Read the model definition and answer for the solid it produces. Units are mm, in the model's axes. Face numbers are marked on the shaded views. A direction names the side the tool comes from. Coordinates: 2 decimals unless noted, no trailing zeros. Write each loop counter-clockwise with the first axis right and the second up, starting at its lowest first coordinate (ties: lowest second). Pieces come first, ordered by that corner, then holes. Notation, with made-up numbers: (47.25, -23.75) -> (67.25, -23.75) arc R19 cw to (67.25, 0.25) -> close; hole circle Ø8 at (0.5, 56). An arc over 180 degrees is marked (long way). Answer as a JSON object with one key per item and string values. Group by question number.
(1) Find section D-D (y = -24). Give the vertices of the cut face in (x, z).
(2) For a pull along Y with two mould halves and no side action, classify the marked faces 1, 2 and 3 as +Y half, -Y half, draft (parallel to the pull), parting line (faces both ways), or undercut.
(3) Flat-ended cylindrical pins translate along their axes: P1, Ø10, axis at y = 10, z = 11, coming from the +X side; P2, Ø3, axis at x = 34, y = 0, coming from the +Z side; P3, Ø6, axis at y = -68.5, z = 5.5, coming from the +X side; P4, Ø1.5, axis at y = -61.5, z = 13, coming from the +X side. Find the tip coordinate at first contact, or state that the pin passes through.
(4) Find section A-A (z = -9). Give the vertices of the cut face in (x, y).
(5) Find section B-B (y = -65.5). Give the vertices of the cut face in (x, z), then the cut area to 3 significant figures.
(6) Straight lines are drawn through the part: L1, parallel to Y at x = 14.5, z = -5; L2, parallel to Y at x = -17, z = 12.5; L3, parallel to Y at x = -17, z = 8.25. For each, find the intervals that lie inside material, in ascending order.
(7) Which of the six approach directions +Z, -Z, +X, -X, +Y, -Y give full straight-line access (tool end or side, diameter ignored) to the marked faces 4, 5, 6, 7 and 8?
(8) Find section C-C (z = 2). Give the vertices of the cut face in (x, y), then the cut area to 3 significant figures.
from build123d import *

# Parameters (mm, degrees)
SKETCH1_R               = 37.5
SKETCH1_R_2             = 29.5
BOSS_EXTRUDE1_DEPTH     = 15
SKETCH2_R               = 32.5
SKETCH2_R_2             = 27.5
CUT_EXTRUDE1_DEPTH      = 7
SKETCH9_R               = 1
CUT_EXTRUDE5_DEPTH      = 15
SKETCH10_R              = 37.5
CUT_EXTRUDE6_DEPTH      = 4
SKETCH7_W               = 45
SKETCH7_H               = 10
BOSS_EXTRUDE3_DEPTH     = 12.5
SKETCH12_R              = 1.5
CUT_EXTRUDE8_DEPTH      = 15
CUT_EXTRUDE9_DEPTH      = 35
CUT_EXTRUDE9_DEPTH_BACK = 35
SKETCH14_W              = 8
SKETCH14_H              = 44.996878368
CUT_EXTRUDE10_DEPTH     = 5


with BuildPart() as part:
    # Sketch1 → Boss-Extrude1 (new body)
    # profile 1 of 2: a face of its own
    with BuildSketch(Plane.XY):
        Circle(SKETCH1_R)
        Circle(SKETCH1_R_2, mode=Mode.SUBTRACT)
    # profile 2 of 2: a face of its own
    with BuildSketch(Plane.XY):
        with BuildLine():
            Line((-22.5, -82.5), (22.5, -82.5))
            Line((22.5, -82.5), (36.841286084, -6.997831068))
            ThreePointArc((36.841286084, -6.997831068), (0, -37.5), (-36.841286084, -6.997831068))
            Line((-36.841286084, -6.997831068), (-22.5, -82.5))
        make_face()
    extrude(amount=BOSS_EXTRUDE1_DEPTH)

    # Sketch2 → Cut-Extrude1 (cut)
    with BuildSketch(Plane(origin=(0, 0, 0), x_dir=(-1, 0, 0), z_dir=(0, 0, -1))):
        Circle(SKETCH2_R)
        Circle(SKETCH2_R_2, mode=Mode.SUBTRACT)
    extrude(amount=-CUT_EXTRUDE1_DEPTH, mode=Mode.SUBTRACT)

    # Sketch9 → Cut-Extrude5 (cut)
    with BuildSketch(Plane.XY.offset(15)):
        with Locations((17, 29.444863729)):
            Circle(SKETCH9_R)
        with Locations((34, 0)):
            Circle(SKETCH9_R)
        with Locations((17, -29.444863729)):
            Circle(SKETCH9_R)
        with Locations((-17, -29.444863729)):
            Circle(SKETCH9_R)
        with Locations((-34, 0)):
            Circle(SKETCH9_R)
        with Locations((-17, 29.444863729)):
            Circle(SKETCH9_R)
    extrude(amount=-CUT_EXTRUDE5_DEPTH, mode=Mode.SUBTRACT)

    # Sketch10 → Cut-Extrude6 (cut)
    with BuildSketch(Plane(origin=(0, 0, 0), x_dir=(-1, 0, 0), z_dir=(0, 0, -1))):
        Circle(SKETCH10_R)
    extrude(amount=-CUT_EXTRUDE6_DEPTH, mode=Mode.SUBTRACT)

    # Sketch7 → Boss-Extrude3 (add)
    with BuildSketch(Plane(origin=(0, 0, 0), x_dir=(-1, 0, 0), z_dir=(0, 0, -1))):
        with Locations((0, -77.5)):
            Rectangle(SKETCH7_W, SKETCH7_H)
        with Locations((0, -42.5)):
            Rectangle(SKETCH7_W, SKETCH7_H)
    extrude(amount=BOSS_EXTRUDE3_DEPTH)

    # Sketch12 → Cut-Extrude8 (cut)
    with BuildSketch(Plane(origin=(0, 0, 0), x_dir=(-1, 0, 0), z_dir=(0, 0, -1))):
        with Locations((-15, -54.5)):
            Circle(SKETCH12_R)
        with Locations((0, -54.5)):
            Circle(SKETCH12_R)
        with Locations((15, -54.5)):
            Circle(SKETCH12_R)
        with Locations((-15, -65.5)):
            Circle(SKETCH12_R)
        with Locations((0, -65.5)):
            Circle(SKETCH12_R)
        with Locations((15, -65.5)):
            Circle(SKETCH12_R)
    extrude(amount=-CUT_EXTRUDE8_DEPTH, mode=Mode.SUBTRACT)

    # Sketch13 → Cut-Extrude9 (cut, two sides: drawn at the far end of the back side and taken through both)
    with BuildSketch(Plane(origin=(0, 0, 0), x_dir=(0, 0, -1), z_dir=(1, 0, 0)).offset(-CUT_EXTRUDE9_DEPTH_BACK)):
        Polygon((-15, -82.5), (-15, -37.5), (-10, -82.5), align=None)
    extrude(amount=CUT_EXTRUDE9_DEPTH + CUT_EXTRUDE9_DEPTH_BACK, mode=Mode.SUBTRACT)

    # Sketch14 → Cut-Extrude10 (cut)
    with BuildSketch(Plane.XY.offset(15)):
        with Locations((-15, -59.998439184)):
            Rectangle(SKETCH14_W, SKETCH14_H)
        with Locations((15, -59.998439184)):
            Rectangle(SKETCH14_W, SKETCH14_H)
        with Locations((0, -59.998439184)):
            Rectangle(SKETCH14_W, SKETCH14_H)
    extrude(amount=-CUT_EXTRUDE10_DEPTH, mode=Mode.SUBTRACT)


solid = part.part
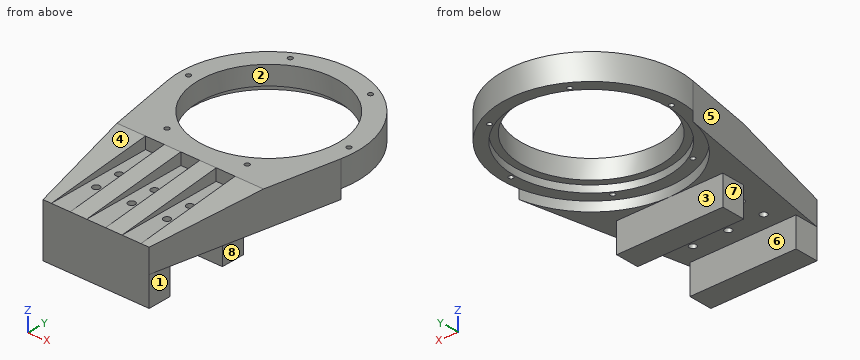
Results below:
{
 "1": {"outline": "(-33.61, 0) -> (-28.81, 0) -> (-28.81, 4) -> (-21.91, 4) -> (-21.91, 7) -> (-17.15, 7) -> (-17.15, 15) -> (-33.61, 15) -> close; (17.15, 7) -> (21.91, 7) -> (21.91, 4) -> (28.81, 4) -> (28.81, 0) -> (33.61, 0) -> (33.61, 15) -> (17.15, 15) -> close"},
 "2": {"face 1": "draft", "face 2": "undercut", "face 3": "+Y half"},
 "3": {"P1": "stops at x = 37.17", "P2": "stops at z = 15", "P3": "stops at x = 25.73", "P4": "stops at x = 26.57"},
 "4": {"outline": "(-22.5, -82.5) -> (22.5, -82.5) -> (22.5, -72.5) -> (-22.5, -72.5) -> close; (-22.5, -47.5) -> (22.5, -47.5) -> (22.5, -37.5) -> (-22.5, -37.5) -> close"},
 "5": {"outline": "(-25.73, 0) -> (-16.5, 0) -> (-16.5, 10) -> (-19, 10) -> (-19, 11.89) -> (-25.73, 11.89) -> close; (-13.5, 0) -> (-1.5, 0) -> (-1.5, 10) -> (-4, 10) -> (-4, 11.89) -> (-11, 11.89) -> (-11, 10) -> (-13.5, 10) -> close; (1.5, 0) -> (13.5, 0) -> (13.5, 10) -> (11, 10) -> (11, 11.89) -> (4, 11.89) -> (4, 10) -> (1.5, 10) -> close; (16.5, 0) -> (25.73, 0) -> (25.73, 11.89) -> (19, 11.89) -> (19, 10) -> (16.5, 10) -> close", "area": "476 mm2"},
 "6": {"L1": "y = -82.5 to -72.5, -47.5 to -37.5", "L2": "y = -37.5 to -30.44, -28.44 to -24.11, 24.11 to 28.44, 30.44 to 33.43", "L3": "y = -82.5 to -30.44, -28.44 to -24.11, 24.11 to 28.44, 30.44 to 33.43"},
 "7": {"face 4": "+Z, +X, -X, -Y", "face 5": "+Z, -Z, -X, -Y", "face 6": "-Z, +X, -X", "face 7": "-Z, -X, +Y, -Y", "face 8": "-Z, +X, +Y, -Y"},
 "8": {"outline": "(-36.84, -7) -> (-22.5, -82.5) -> (22.5, -82.5) -> (36.84, -7) arc R37.5 cw to start; hole circle Ø3 at (-15, -65.5); hole circle Ø3 at (-15, -54.5); hole circle Ø3 at (0, -65.5); hole circle Ø3 at (0, -54.5); hole circle Ø3 at (15, -65.5); hole circle Ø3 at (15, -54.5)", "area": "2,750 mm2"}
}
